```python
from build123d import *

# Parameters (mm, degrees)
EXTRUDE_THIN1_DEPTH = 36.7
SKETCH4_W           = 21.133468013
SKETCH4_H           = 40.04871341
CUT_EXTRUDE2_DEPTH  = 54.616609778
SKETCH5_R           = 4.5
CUT_EXTRUDE3_DEPTH  = 54.616609778
SKETCH6_R           = 2.915
CUT_EXTRUDE4_DEPTH  = 54.616609778
SKETCH7_R           = 0.75
CUT_EXTRUDE5_DEPTH  = 54.616609778
SKETCH8_R           = 1.25
CUT_EXTRUDE6_DEPTH  = 54.616609778
SKETCH9_W           = 36.7
SKETCH9_H           = 7.475480679
CUT_EXTRUDE7_DEPTH  = 54.616609778


with BuildPart() as part:
    # Sketch3 → Extrude-Thin1 (new body)
    with BuildSketch(Plane(origin=(0, 0, 0), x_dir=(0, 0, -1), z_dir=(1, 0, 0))):
        Polygon((0, 0), (0, -26.128965265), (24.534239686, -26.128965265), (24.534239686, -30.428965265), (-4.3, -30.428965265), (-4.3, 0), align=None)
    extrude(amount=-EXTRUDE_THIN1_DEPTH)

    # Sketch4 → Cut-Extrude2 (cut, through all)
    with BuildSketch(Plane(origin=(0, 0, 0), x_dir=(1, 0, 0), z_dir=(0, 1, 0))):
        with Locations((-37.126734007, 19.219871441)):
            Rectangle(SKETCH4_W, SKETCH4_H)
    extrude(amount=-CUT_EXTRUDE2_DEPTH, mode=Mode.SUBTRACT)

    # Sketch5 → Cut-Extrude3 (cut, through all)
    with BuildSketch(Plane.XY):
        with Locations((-11.4, -20.118965265)):
            Circle(SKETCH5_R)
    extrude(amount=CUT_EXTRUDE3_DEPTH, mode=Mode.SUBTRACT)

    # Sketch6 → Cut-Extrude4 (cut, through all)
    with BuildSketch(Plane.XY):
        with Locations((-22.1, -20.118965265)):
            Circle(SKETCH6_R)
    extrude(amount=CUT_EXTRUDE4_DEPTH, mode=Mode.SUBTRACT)

    # Sketch7 → Cut-Extrude5 (cut, through all)
    with BuildSketch(Plane.XY):
        with Locations((-32.75, -11.248965265)):
            Circle(SKETCH7_R)
        with Locations((-32.75, -28.998965265)):
            Circle(SKETCH7_R)
    extrude(amount=CUT_EXTRUDE5_DEPTH, mode=Mode.SUBTRACT)

    # Sketch8 → Cut-Extrude6 (cut, through all)
    with BuildSketch(Plane(origin=(0, 0, 0), x_dir=(1, 0, 0), z_dir=(0, 1, 0))):
        with Locations(Location((-19.027267825, 11.350303501, 0), (0, 0, 270))):
            Circle(SKETCH8_R)
        with Locations(Location((-19.027267825, 19.701887491, 0), (0, 0, 270))):
            Circle(SKETCH8_R)
        with Locations(Location((-6.907228252, 11.350303501, 0), (0, 0, 270))):
            Circle(SKETCH8_R)
        with Locations(Location((-6.45179676, 19.701887491, 0), (0, 0, 270))):
            Circle(SKETCH8_R)
    extrude(amount=-CUT_EXTRUDE6_DEPTH, mode=Mode.SUBTRACT)

    # Sketch9 → Cut-Extrude7 (cut, through all)
    with BuildSketch(Plane.XY):
        with Locations((-18.35, -3.73774034)):
            Rectangle(SKETCH9_W, SKETCH9_H)
    extrude(amount=CUT_EXTRUDE7_DEPTH, mode=Mode.SUBTRACT)


solid = part.part
```
Input: part model. Units: mm. Frame: model coordinates. A direction names the side the tool comes from. Give positions to 0.01 mm unless a question says otherwise; leave off trailing zeros. Write each loop counter-clockwise with the first axis right and the second up, starting at its lowest first coordinate (ties: lowest second). Pieces come first, ordered by that corner, then holes. Notation, with made-up numbers: (77, 78) - (115, 78) arc R14 cw to (115, 84) - close; hole circle Ø3 at (10.5, -2). An arc over 180 degrees is marked (long way). Write item = value, one per line. Start each with the question number.
1) Pin query (flat end, axial travel): pin 1 (6 mm diameter, centred on x = -15.5, y = -17, fed in from -Z); pin 2 (3 mm diameter, centred on x = -6.45, z = -19.7, fed in from +Y); pin 3 (3 mm diameter, centred on x = -32.5, y = -22, fed in from -Z). Return the tip coordinate at first contact, or that it passes through.
2) Draft query along Y for faces 1 (the face through (-14.72, -17.08, 2.12)), 2 (the face through (-20.755, -22.705, 2.12)), 3 (the face through (-18, -19, 4.3)), 4 (the face through (-13, -26.129, -12)). Return one class per face: pulls with the +Y half, pulls with the -Y half, needs draft (parallel to the pull), parting line crosses it, or undercut.
3) Material intervals for L1, parallel to Y at x = -32.75, z = 1.75; L2, parallel to X at y = -22.75, z = 0.25; L3, parallel to Z at x = -34, y = -13.25, sorted ascending. Write a range as [from, to].
4) Cut plane D-D (y = -10). Return loops of the section in (x, z).
5) Cut plane C-C (z = -11.5). Return loops of the section in (x, y).
6) Cut plane A-A (x = -11.4). Return loops of the section in (y, z), and give its area (3 significant figures).
7) Cut plane B-B (x = -32.75). Return loops of the section in (y, z).
8) Reachability of faces 5 (the face through (-13, -15, 0)), 6 (the face through (-26.56, -27, -10)), 7 (the face through (-6.931, -28.249, -18.547)) from +Z, -Z, +X, -X, +Y, -Y: full face, straight path, thin tool, end or side. Return the list, or none.
Answers follow:
q1.pin_1 = 0
q1.pin_2 = -26.13
q1.pin_3 = 0.8
q2.face_1 = undercut
q2.face_2 = undercut
q2.face_3 = needs draft
q2.face_4 = pulls with the +Y half
q3.L1 = [-30.43, -29.75], [-28.25, -12], [-10.5, -7.48]
q3.L2 = [-26.56, -23.35], [-20.85, -15.05], [-7.75, 0]
q3.L3 = [0.8, 4.3]
q4.outline = (-36.7, 0.8) - (-26.56, 0.8) - (-26.56, 0) - (0, 0) - (0, 4.3) - (-36.7, 4.3) - close
q5.outline = (-26.56, -30.43) - (-20.27, -30.43) - (-20.27, -26.13) - (-26.56, -26.13) - close; (-17.79, -30.43) - (-8.15, -30.43) - (-8.15, -26.13) - (-17.79, -26.13) - close; (-5.67, -30.43) - (0, -30.43) - (0, -26.13) - (-5.67, -26.13) - close
q6.outline = (-30.43, -24.53) - (-26.13, -24.53) - (-26.13, 0) - (-24.62, 0) - (-24.62, 4.3) - (-30.43, 4.3) - close; (-15.62, 0) - (-7.48, 0) - (-7.48, 4.3) - (-15.62, 4.3) - close
q6.area = 165 mm^2
q7.outline = (-30.43, 0.8) - (-29.75, 0.8) - (-29.75, 4.3) - (-30.43, 4.3) - close; (-28.25, 0.8) - (-12, 0.8) - (-12, 4.3) - (-28.25, 4.3) - close; (-10.5, 0.8) - (-7.48, 0.8) - (-7.48, 4.3) - (-10.5, 4.3) - close
q8.face_5 = -Z, +X, -X, +Y
q8.face_6 = -Z, -X, +Y, -Y
q8.face_7 = +Y, -Y
